Verification items for this drawing (mm, ordinates from the low corner). A direction names the side the tool comes from. Give positions to 0.01 mm unless a question says otherwise; leave off trailing zeros. Order: outer loops, then holes, each group sorted by start corner. A loop starts at its lowest first (then second) coordinate and runs counter-clockwise, first axis right, second up. Notation, with made-up numbers: (78.25, -32.5) - (90.25, -32.5) arc R34 ccw to (90.25, 6.5) - close; hole circle Ø4 at (67.5, -36.75). An arc over 180 degrees is marked (long way). Put each result on its own line as item: value. Start each with the question number.
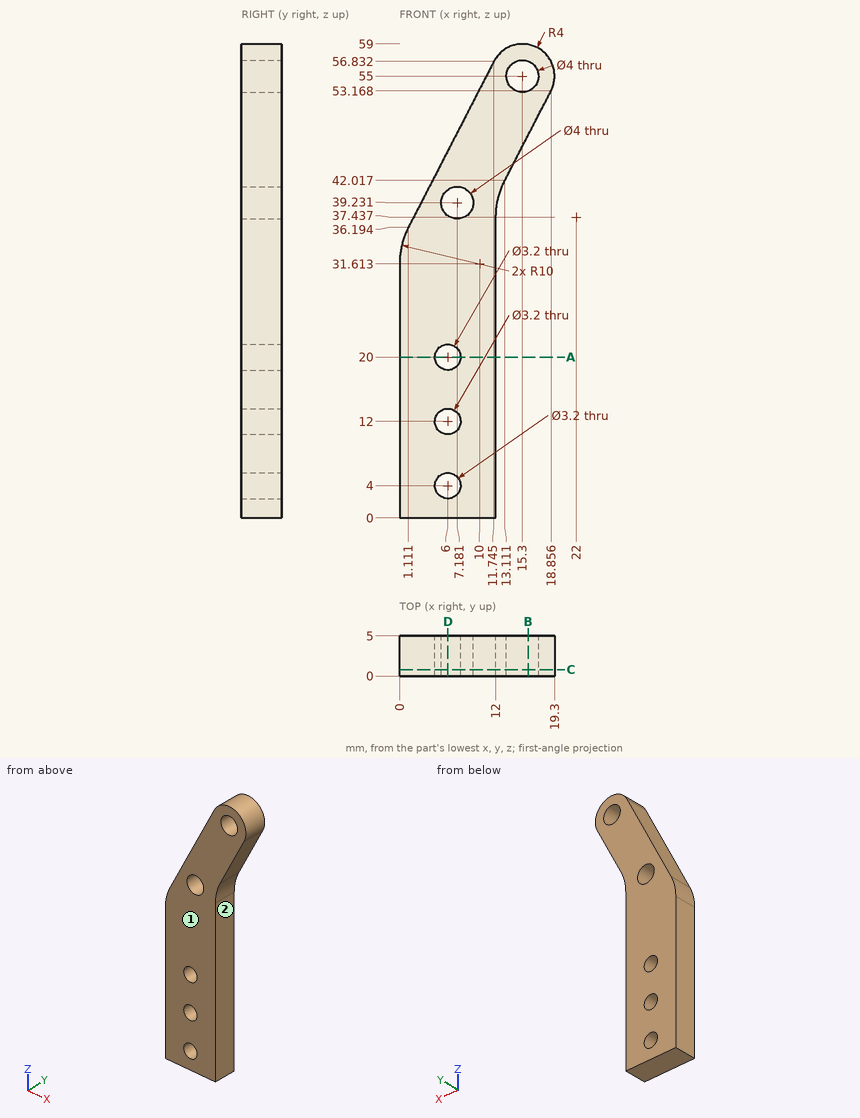
Item 1: Set-up check for the marked faces 1 and 2: record each of +Z, -Z, +X, -X, +Y, -Y from which the full face is reachable in a straight line by a thin tool's end or side.
Item 2: Gauge pin test, flat ends, axial feed: pin 1 Ø1.9 at (x, z) = (6, 12) entering from -Y; pin 2 Ø3 at (y, z) = (3.5, 24) entering from +X; pin 3 Ø1.5 at (x, y) = (2, 1) entering from +Z (1 decimal). Record the tip position at first contact, or that the pin passes through.
Item 3: Cross-section at A-A (z = 20). Enter the section's corners in (x, y), and give its area (3 significant figures).
Item 4: Cross-section at D-D (x = 6). Enter the section's corners in (y, z) (1 decimal).
Item 5: Cross-section at B-B (x = 16). Enter the section's corners in (y, z) (1 decimal).
Item 6: Cross-section at C-C (y = 0.8). Enter the section's corners in (x, z) (1 decimal).
Item 7: Thickness scan on line 1 along X through (y, z) = (1.9, 4); line 2 along Z through (x, y) = (7.25, 4.55) (1 decimal); line 3 along Z through (x, y) = (6.25, 1.7) (1 decimal). Record the ranges inside material, lowest first.
Recorded:
1. face 1: +Z, -Z, +X, -X, -Y
1. face 2: -Z, +X, +Y, -Y
2. pin 1: passes through
2. pin 2: stops at x = 12
2. pin 3: stops at z = 39.4
3. outline: (0, 0) - (4.4, 0) - (4.4, 5) - (0, 5) - close; (7.6, 0) - (12, 0) - (12, 5) - (7.6, 5) - close
3. area: 44.0 mm^2
4. outline: (0, 0) - (5, 0) - (5, 2.4) - (0, 2.4) - close; (0, 5.6) - (5, 5.6) - (5, 10.4) - (0, 10.4) - close; (0, 13.6) - (5, 13.6) - (5, 18.4) - (0, 18.4) - close; (0, 21.6) - (5, 21.6) - (5, 37.6) - (0, 37.6) - close; (0, 40.8) - (5, 40.8) - (5, 45.7) - (0, 45.7) - close
5. outline: (0, 47.6) - (5, 47.6) - (5, 53.1) - (0, 53.1) - close; (0, 56.9) - (5, 56.9) - (5, 58.9) - (0, 58.9) - close
6. outline: (0, 0) - (12, 0) - (12, 37.4) arc R10 cw to (13.1, 42) - (18.9, 53.2) arc R4 ccw to (11.7, 56.8) - (1.1, 36.2) arc R10 ccw to (0, 31.6) - close; hole circle Ø3.2 at (6, 4); hole circle Ø3.2 at (6, 12); hole circle Ø3.2 at (6, 20); hole circle Ø4 at (7.2, 39.2); hole circle Ø4 at (15.3, 55)
7. line 1: x = 0 to 4.4, 7.6 to 12
7. line 2: z = 0 to 3, 5 to 11, 13 to 19, 21 to 37.2, 41.2 to 48.1
7. line 3: z = 0 to 2.4, 5.6 to 10.4, 13.6 to 18.4, 21.6 to 37.5, 41 to 46.2
